Work out the finished part from the listing and answer in its coordinate system (mm). A direction names the side the tool comes from. Round coordinates to 2 decimals unless told otherwise and drop trailing zeros. Order: outer loops, then holes, each group sorted by start corner. A loop starts at its lowest first (then second) coordinate and runs counter-clockwise, first axis right, second up. Notation, with made-up numbers: M 47.5,-27 L 63.5,-27 A21 ccw 63.5,-20 Z; hole C 85.25,-12 d7. An arc over 180 degrees is marked long. Answer as a JSON object with one key per item and string values. Group by question number.
from build123d import *
from build123d.topology import SkipClean

# Parameters (mm, degrees)
SKETCH_1_W                = 76.6
SKETCH_1_H                = 23.8
EXTRUDE_1_DEPTH           = 31.899999991
HOLE_WIZARD_M4_1_D        = 3.3
HOLE_WIZARD_M4_1_DEPTH    = 10.1
HOLE_WIZARD_M4_1_TIP      = 0.991420021
SKETCH_5_W                = 23.8
SKETCH_5_H                = 2.281370048
EXTRUDE_2_DEPTH           = 2.994
SKETCH_6_W                = 76.6
SKETCH_6_H                = 2.281370048
EXTRUDE_3_DEPTH           = 2.944
CUT_EXTRUDE_START         = -2.994
SKETCH_7_W                = 26.992148155
SKETCH_7_H                = 47.339562986
CUT_EXTRUDE_1_DEPTH       = 2.994
EXTRUDE_4_DEPTH           = 10
HOLE_WIZARD_3_D           = 6.6
HOLE_WIZARD_3_CBORE_D     = 11
HOLE_WIZARD_3_CBORE_DEPTH = 6.8
SKETCH_21_R               = 3.3
CUT_EXTRUDE_6_DEPTH       = 67.034934903
MM_2_D                    = 4
MM_2_DEPTH                = 5
MM_2_TIP                  = 1.201721238
CUT_EXTRUDE_7_DEPTH       = 5
SKETCH_26_W               = 46.053862543
SKETCH_26_H               = 10
CUT_EXTRUDE_8_DEPTH       = 76.924939501
CUT_EXTRUDE_9_DEPTH       = 67.034934903
SKETCH_29_R               = 1
CUT_EXTRUDE_10_DEPTH      = 2.281370048
EXTRUDE_START             = 4
EXTRUDE_5_DEPTH           = 4
CUT_EXTRUDE_11_DEPTH      = 0.5
EXTRUDE_6_DEPTH           = 0.440630619
CUT_EXTRUDE_12_DEPTH      = 28.181370038
SKETCH_35_W               = 0.294839433
SKETCH_35_H               = 10
CUT_EXTRUDE_13_DEPTH      = 100.471808588
CHAMFER_1_SIZE            = 2
HOLE_WIZARD_4_D           = 4.5
HOLE_WIZARD_4_CBORE_D     = 8
HOLE_WIZARD_4_CBORE_DEPTH = 25
CUT_EXTRUDE_14_DEPTH      = 67.233425798
CUT_EXTRUDE_15_DEPTH      = 6.281370048


with BuildPart() as part:
    # 草图1 → 凸台-拉伸1 (new body)
    with BuildSketch(Plane(origin=(0, 0, 0), x_dir=(1, 0, 0), z_dir=(0, 1, 0))):
        Rectangle(SKETCH_1_W, SKETCH_1_H)
    extrude(amount=-EXTRUDE_1_DEPTH)

    # M4 螺纹孔1
    with Locations(Plane(origin=(0, 0, -5.4), x_dir=(0, 0, 1), z_dir=(0, 1, 0))):
        with Locations((0, 0)):
            Hole(HOLE_WIZARD_M4_1_D / 2, depth=HOLE_WIZARD_M4_1_DEPTH)
            with Locations((0, 0, -(HOLE_WIZARD_M4_1_DEPTH + HOLE_WIZARD_M4_1_TIP / 2))):  # 118° drill point
                Cone(0, HOLE_WIZARD_M4_1_D / 2, HOLE_WIZARD_M4_1_TIP, mode=Mode.SUBTRACT)

    # 草图5 → 凸台-拉伸2 (add)
    with BuildSketch(Plane.ZY.offset(38.3)):
        with Locations((0, 1.140685024)):
            Rectangle(SKETCH_5_W, SKETCH_5_H)
    extrude(amount=-EXTRUDE_2_DEPTH)

    # 草图6 → 凸台-拉伸3 (add)
    with BuildSketch(Plane(origin=(0, 0, -11.9), x_dir=(-1, 0, 0), z_dir=(0, 0, -1))):
        with Locations((0, 1.140685024)):
            Rectangle(SKETCH_6_W, SKETCH_6_H)
    extrude(amount=-EXTRUDE_3_DEPTH)

    # 草图7 → 切除-拉伸1 (cut)
    with BuildSketch(Plane(origin=(38.3, 0, 0), x_dir=(0, 0, -1), z_dir=(1, 0, 0)).offset(CUT_EXTRUDE_START)):
        with Locations((-1.596074077, -8.230218498)):
            Rectangle(SKETCH_7_W, SKETCH_7_H)
    extrude(amount=CUT_EXTRUDE_1_DEPTH, mode=Mode.SUBTRACT)

    # 草图9 → 大小mm 暗销孔1 (revolve, cut)
    with BuildSketch(Plane(origin=(17.4625, 0, -4.384), x_dir=(0, 0, 1), z_dir=(1, 0, 0))):
        Polygon((0, 0), (0, 5.96137699), (1.6, 5), (1.6, 0), align=None)
    mm_1 = revolve(axis=Axis((17.4625, 6.35, -4.384), (0, -1, 0)), mode=Mode.SUBTRACT)

    # 镜向3: 大小mm 暗销孔1 across plane
    add(mm_1.mirror(Plane(origin=(0, 0, 0), x_dir=(0, 0, 1), z_dir=(1, 0, 0))), mode=Mode.SUBTRACT)

    # 草图16 → 凸台-拉伸4 (add)
    with BuildSketch(Plane.XZ.offset(31.899999991)):
        Polygon((-38.3, 6.921881597), (-55.247298311, -11.9), (-38.3, -11.9), align=None)
        Polygon((-33.817682057, 11.9), (-20.311621392, 26.9), (35.306, 26.9), (35.306, 11.9), align=None)
    extrude(amount=-EXTRUDE_4_DEPTH)

    # 打孔尺寸(%根据)内六角圆柱头螺钉的类型3 (through all)
    with Locations(Plane(origin=(-14.255841028, -21.899999991, 19.4), x_dir=(1, 0, 0), z_dir=(0, 1, 0))):
        with Locations((0, 0), (15, 0), (35, 0)):
            CounterBoreHole(HOLE_WIZARD_3_D / 2, HOLE_WIZARD_3_CBORE_D / 2, HOLE_WIZARD_3_CBORE_DEPTH)

    # 草图21 → 切除-拉伸6 (cut, through all)
    with BuildSketch(Plane(origin=(0, -21.899999991, 0), x_dir=(1, 0, 0), z_dir=(0, 1, 0))):
        with Locations(Location((-44.3, 5.9, 0), (0, 0, 180))):
            Circle(SKETCH_21_R)
    extrude(amount=-CUT_EXTRUDE_6_DEPTH, mode=Mode.SUBTRACT)

    # 大小mm 暗销孔2
    with Locations(Plane(origin=(10.744158972, -31.899999991, 9.4), x_dir=(0, 0, -1), z_dir=(0, -1, 0))):
        with Locations((0, 0)):
            Hole(MM_2_D / 2, depth=MM_2_DEPTH)
            with Locations((0, 0, -(MM_2_DEPTH + MM_2_TIP / 2))):  # 118° drill point
                Cone(0, MM_2_D / 2, MM_2_TIP, mode=Mode.SUBTRACT)

    # 草图25 → 切除-拉伸7 (cut)
    with BuildSketch(Plane.XZ.offset(31.899999991)):
        with BuildLine():
            Line((-9.755841028, 11.4), (-8.755841028, 11.4))
            ThreePointArc((-8.755841028, 11.4), (-6.755841028, 9.4), (-8.755841028, 7.4))
            Line((-8.755841028, 7.4), (-9.755841028, 7.4))
            ThreePointArc((-9.755841028, 7.4), (-11.755841028, 9.4), (-9.755841028, 11.4))
        make_face()
    extrude(amount=-CUT_EXTRUDE_7_DEPTH, mode=Mode.SUBTRACT)

    # 草图26 → 切除-拉伸8 (cut, through all)
    with BuildSketch(Plane(origin=(-24.593701474, 0, 22.144268272), x_dir=(0.6691306063588817, 0, 0.7431448254773731), z_dir=(-0.7431448254773731, 0, 0.6691306063588817))):
        with Locations((-11.827706241, -26.899999991)):
            Rectangle(SKETCH_26_W, SKETCH_26_H)
    extrude(amount=CUT_EXTRUDE_8_DEPTH, mode=Mode.SUBTRACT)

    # 草图27 → 切除-拉伸9 (cut, through all)
    with BuildSketch(Plane.XZ.offset(21.899999991)):
        Polygon((-38.3, 6.921881597), (-33.817682057, 11.9), (-38.3, 11.9), align=None)
    extrude(amount=-CUT_EXTRUDE_9_DEPTH, mode=Mode.SUBTRACT)

    # 草图29 → 切除-拉伸10 (cut)
    with BuildSketch(Plane(origin=(0, 2.281370048, 0), x_dir=(1, 0, 0), z_dir=(0, 1, 0))):
        with Locations((-35.306, 8.956)):
            Circle(SKETCH_29_R)
    extrude(amount=-CUT_EXTRUDE_10_DEPTH, mode=Mode.SUBTRACT)

    # 草图31 → 凸台-拉伸5 (add)
    with SkipClean():  # the faces are left unmerged after this step: merging them gives an invalid solid
        with BuildSketch(Plane(origin=(0, 2.281370048, 0), x_dir=(1, 0, 0), z_dir=(0, 1, 0)).offset(EXTRUDE_START)):
            with BuildLine():
                Line((-34.306, 8.956), (35.306, 8.956))
                Line((35.306, 8.956), (35.306, 11.9))
                Line((35.306, 11.9), (-38.3, 11.9))
                Line((-38.3, 11.9), (-38.3, -6.921881597))
                Line((-38.3, -6.921881597), (-35.306, -10.247055466))
                Line((-35.306, -10.247055466), (-35.306, 7.956))
                ThreePointArc((-35.306, 7.956), (-36.013106781, 9.663106781), (-34.306, 8.956))
            make_face()
        extrude(amount=-EXTRUDE_5_DEPTH)

    # 草图32 → 切除-拉伸11 (cut)
    with SkipClean():  # the faces are left unmerged after this step: merging them gives an invalid solid
        with BuildSketch(Plane(origin=(-24.593701474, 0, 22.144268272), x_dir=(0.6691306063588817, 0, 0.7431448254773731), z_dir=(-0.7431448254773731, 0, 0.6691306063588817))):
            Polygon((-23.813531784, -21.899999991), (-45.811081642, -21.899999991), (-45.811081642, -31.899999991), (7.49870663, -31.899999991), (7.49870663, -21.899999991), (-11.951824765, -21.899999991), (-11.951824765, 0), (-16.009278942, 0), (-16.009278942, 6.281370048), (-23.813531784, 6.281370048), align=None)
        extrude(amount=-CUT_EXTRUDE_11_DEPTH, mode=Mode.SUBTRACT)

    # 草图33 → 凸台-拉伸6 (add)
    with SkipClean():  # the faces are left unmerged after this step: merging them gives an invalid solid
        with BuildSketch(Plane(origin=(-24.222129061, 0, 21.809702968), x_dir=(0.6691306063588818, 0, 0.743144825477373), z_dir=(-0.743144825477373, 0, 0.6691306063588818))):
            Polygon((-45.36087962, -21.899999991), (-45.36087962, -31.899999991), (6.849670289, -31.899999991), (6.849670289, -21.899999991), (-13.334820655, -21.899999991), (-13.334820655, 0), (-16.564585199, 0), (-16.564585199, 6.281370048), (-21.03904799, 6.281370048), (-21.03904799, -21.899999991), align=None)
        extrude(amount=EXTRUDE_6_DEPTH)

    # 草图34 → 切除-拉伸12 (cut)
    with SkipClean():  # the faces are left unmerged after this step: merging them gives an invalid solid
        with BuildSketch(Plane(origin=(0, 6.281370048, 0), x_dir=(1, 0, 0), z_dir=(0, 1, 0))):
            Polygon((-38.3, -6.174643322), (-38.3, -6.833155448), (-38.627452364, -6.469482755), align=None)
            Polygon((-33.144865692, -11.9), (-33.737792674, -11.9), (-33.472318056, -12.194839433), align=None)
        extrude(amount=-CUT_EXTRUDE_12_DEPTH, mode=Mode.SUBTRACT)

    # 草图35 → 切除-拉伸13 (cut, through all)
    with SkipClean():  # the faces are left unmerged after this step: merging them gives an invalid solid
        with BuildSketch(Plane(origin=(35.306, 0, 0), x_dir=(0, 0, -1), z_dir=(1, 0, 0))):
            with Locations((-27.047419717, -26.899999991)):
                Rectangle(SKETCH_35_W, SKETCH_35_H)
        extrude(amount=-CUT_EXTRUDE_13_DEPTH, mode=Mode.SUBTRACT)

    # 倒角1
    # the kernel refuses this chamfer: 2 mm, written as the material it takes off along each edge
    with BuildSketch(Plane(origin=(-54.901934311, -16.756634015, -11.605160567), x_dir=(0.7244655223975905, 0, -0.6893110378176068), z_dir=(0, -1, 0))) as chamfer_1_piece_1:
        Polygon((CHAMFER_1_SIZE * 0.999621916911, CHAMFER_1_SIZE * 0.0274958766106), (-CHAMFER_1_SIZE * 0.0274958766106, CHAMFER_1_SIZE * 0.999621916911), (0, 0), align=None)
    extrude(amount=20.286731952, mode=Mode.SUBTRACT)
    with BuildSketch(Plane(origin=(-35.633452364, 0, 9.794656625), x_dir=(-0.6893110378176083, 0, -0.7244655223975892), z_dir=(0, 1, 0))) as chamfer_1_piece_2:
        Polygon((CHAMFER_1_SIZE * 0.999621916911, -CHAMFER_1_SIZE * 0.0274958766106), (-CHAMFER_1_SIZE * 0.0274958766106, -CHAMFER_1_SIZE * 0.999621916911), (0, 0), align=None)
    extrude(amount=11.424736024, mode=Mode.SUBTRACT)

    # 打孔尺寸(%根据)内六角圆柱头螺钉的类型4 (through all)
    with Locations(Plane(origin=(12.5, -31.899999991, -4.384), x_dir=(0, 0, -1), z_dir=(0, -1, 0))):
        with Locations((0, 0)):
            hole_wizard_4 = CounterBoreHole(HOLE_WIZARD_4_D / 2, HOLE_WIZARD_4_CBORE_D / 2, HOLE_WIZARD_4_CBORE_DEPTH)

    # 镜向4: 打孔尺寸(%根据)内六角圆柱头螺钉的类型4 across plane
    add(hole_wizard_4.mirror(Plane(origin=(0, 0, 0), x_dir=(0, 0, 1), z_dir=(1, 0, 0))), mode=Mode.SUBTRACT)

    # 草图39 → 切除-拉伸14 (cut, through all)
    with BuildSketch(Plane(origin=(0, -21.899999991, 0), x_dir=(1, 0, 0), z_dir=(0, 1, 0))):
        Polygon((-53.470328078, 11.9), (-53.470328078, 10.015200769), (-53.563673098, 10.118870916), align=None)
    extrude(amount=-CUT_EXTRUDE_14_DEPTH, mode=Mode.SUBTRACT)

    # 草图40 → 切除-拉伸15 (cut)
    with BuildSketch(Plane(origin=(0, 6.281370048, 0), x_dir=(1, 0, 0), z_dir=(0, 1, 0))):
        Polygon((-38.3, -6.837514338), (-35.306, -6.837514338), (-35.306, -8.395663323), (-36.971713577, -8.308366973), align=None)
    extrude(amount=-CUT_EXTRUDE_15_DEPTH, mode=Mode.SUBTRACT)


solid = part.part
Item 1: Find section D-D (z = 19.4). Give the vertices of the cut face in (x, y).
Item 2: Find section B-B (x = 22). Give the vertices of the cut face in (y, z), and give its area (3 significant figures).
Item 3: Each of these flat-tipped pins is pushed along its axis until it touches: pin 1 (4 mm diameter, centred on x = -10, z = -5.5, fed in from +Y); pin 2 (3 mm diameter, centred on x = 10.74, z = 9.4, fed in from -Y); pin 3 (10.5 mm diameter, centred on x = -44.3, z = -5.9, fed in from +Y); pin 4 (8.5 mm diameter, centred on x = -14.26, z = 19.4, fed in from -Y). Where does it stop, or does it pass through?
Item 4: Consider L1, parallel to X at y = -10.5, z = -2; L2, parallel to X at y = -25.5, z = 16; L3, parallel to Z at x = 21, y = 2.5. Determine where each line is inside the solid, lowest interval first.
Item 5: Find section C-C (y = -1.5). Give the vertices of the cut face in (x, z).
Item 6: A tool of negligible diameter and unlimited length cuts with its end or side. For faces 1 (the flat face through (1, -28.7, 23)), 2 (the flat face through (-37, 3, 6.838)), 3 (the cylindrical face through (-13.826, -30.322, 16.128)), 4 (the flat face through (10.8, -6.9, -6.1)), from which of +Z, -Z, +X, -X, +Y, -Y can it reach the whole face along a straight path? Write none if from no direction.
Item 7: The mould has two halves that part along X. Classify faces 5 (the cylindrical face through (-15.873, -19.575, -6.534)), 6 (the flat face through (-38.3, -8, -3)), 7 (the flat face through (-6, -31.9, 3)), 8 (the cylindrical face through (-15.45, -25.25, 24.77)): +X half, -X half, draft (parallel to the pull), parting line (faces both ways), or undercut.
Item 8: Find section A-A (y = -21). Give the vertices of the cut face in (x, z), and give its area (3 significant figures).
Responses:
{
 "1": {"outline": "M -26.98,-31.9 L -17.56,-31.9 L -17.56,-28.7 L -19.76,-28.7 L -19.76,-21.9 L -26.98,-21.9 Z; M -10.96,-31.9 L -2.56,-31.9 L -2.56,-28.7 L -4.76,-28.7 L -4.76,-21.9 L -8.76,-21.9 L -8.76,-28.7 L -10.96,-28.7 Z; M 4.04,-31.9 L 17.44,-31.9 L 17.44,-28.7 L 15.24,-28.7 L 15.24,-21.9 L 6.24,-21.9 L 6.24,-28.7 L 4.04,-28.7 Z; M 24.04,-31.9 L 35.31,-31.9 L 35.31,-21.9 L 26.24,-21.9 L 26.24,-28.7 L 24.04,-28.7 Z"},
 "2": {"outline": "M -31.9,-11.9 L 6.28,-11.9 L 6.28,-8.96 L 0,-8.96 L 0,11.9 L -21.9,11.9 L -21.9,14.05 L -28.7,14.05 L -28.7,16.35 L -31.9,16.35 Z; M -31.9,22.45 L -28.7,22.45 L -28.7,24.75 L -21.9,24.75 L -21.9,26.9 L -31.9,26.9 Z", "area": "835 mm^2"},
 "3": {"pin 1": "stops at y = 0", "pin 2": "stops at y = -26.6", "pin 3": "stops at y = -21.9", "pin 4": "stops at y = -31.9"},
 "4": {"L1": "x = -38.3 to -15.71, -9.29 to 9.29, 15.71 to 35.31", "L2": "x = -30.05 to -18.58, -9.93 to -3.58, 5.07 to 16.42, 25.07 to 35.31", "L3": "z = -11.9 to -8.96"},
 "5": {"outline": "M -38.3,-11.9 L 35.31,-11.9 L 35.31,11.9 L -33.74,11.9 L -38.3,6.83 Z; hole C -17.46,-4.38 d3.2; hole C -12.5,-4.38 d4.5; hole C 0,-5.4 d3.3; hole C 12.5,-4.38 d4.5; hole C 17.46,-4.38 d3.2"},
 "6": {"face 1": "+Y", "face 2": "+Z, +X, -X, +Y", "face 3": "+Y, -Y", "face 4": "-Y"},
 "7": {"face 5": "undercut", "face 6": "-X half", "face 7": "draft", "face 8": "undercut"},
 "8": {"outline": "M -38.3,-11.9 L 35.31,-11.9 L 35.31,11.9 L -33.74,11.9 L -38.3,6.83 Z; hole C -12.5,-4.38 d8; hole C 12.5,-4.38 d8", "area": "1,640 mm^2"}
}
